Here's how the part is built. I have some questions about the finished solid (model axes, mm). Round coordinates to 2 decimals unless told otherwise and drop trailing zeros. Write each loop counter-clockwise with the first axis right and the second up, starting at its lowest first coordinate (ties: lowest second). Pieces come first, ordered by that corner, then holes. Notation, with made-up numbers: (56, -13) -> (75, -13) arc R21 ccw to (75, 11) -> close; hole circle Ø6 at (-36.75, -21). An arc over 180 degrees is marked (long way). Answer in a Markdown table with one row per item. Add a question column.
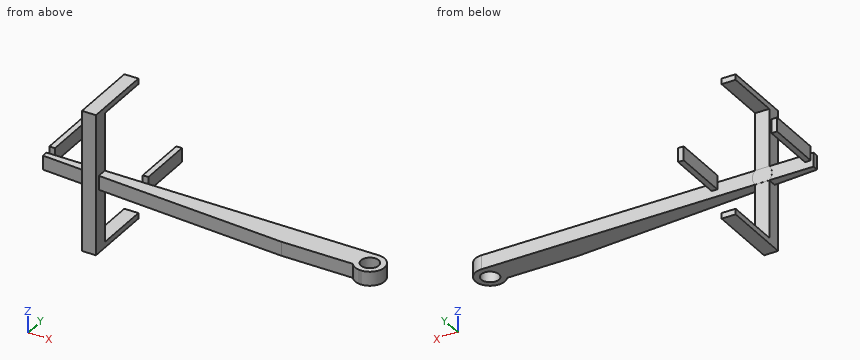
from build123d import *

# Parameters (mm, degrees)
SKETCH1_R             = 6.3
BOSS_EXTRUDE2_DEPTH   = 10
BODY_MOVE_COPY1_ANGLE = 90
BOSS_EXTRUDE4_DEPTH   = 10.5
BOSS_EXTRUDE5_DEPTH   = 0.05
SKETCH5_W             = 4
SKETCH5_H             = 39.958
BOSS_EXTRUDE6_DEPTH   = 10
SKETCH6_W             = 4
SKETCH6_H             = 40
BOSS_EXTRUDE7_DEPTH   = 10


# Read off the part's stored shape, not the designer's step: Boss-Extrude5
with BuildPart() as part:
    # Sketch1 → Boss-Extrude2 (new body)
    with BuildSketch(Plane.XY):
        with BuildLine():
            ThreePointArc((10.5, 0), (0, 10.5), (-10.5, 0))
            Line((-10.5, 0), (-10.5, -236.5))
            Line((-10.5, -236.5), (-6.3, -236.5))
            Line((-6.3, -236.5), (6.3, -59.125))
            Line((6.3, -59.125), (6.3, -8.4))
            ThreePointArc((6.3, -8.4), (9.035151526, -5.349395938), (10.394563839, -1.484265))
            Line((10.394563839, -1.484265), (10.5, 0))
        make_face()
        Circle(SKETCH1_R, mode=Mode.SUBTRACT)
    extrude(amount=BOSS_EXTRUDE2_DEPTH)


with BuildPart() as part_1:
    # Body-Move_Copy1: moved
    add(part.part.rotate(Axis((-34.8, -34.75, 0), (0, 0, -1)), BODY_MOVE_COPY1_ANGLE))


with BuildPart() as part_2:
    # Body-Move_Copy2: moved
    add(part_1.part.moved(Location((0, 69.6, 0))))

    # Sketch3 → Boss-Extrude4 (add)
    with BuildSketch(Plane(origin=(0, 0, 0), x_dir=(1, 0, 0), z_dir=(0, 1, 0))):
        Polygon((-195.05, 45), (-205.05, 45), (-205.05, -45), (-205.05, -55), (-195.05, -55), (-195.05, -5), align=None)
    extrude(amount=BOSS_EXTRUDE4_DEPTH)

    # Boss-Extrude5 outline → Boss-Extrude5 (add)
    with BuildSketch(Plane(origin=(0, 10.55, 0), x_dir=(1, 0, 0), z_dir=(0, 1, 0))):
        with BuildLine():
            ThreePointArc((-195.151020514, -10), (-193.05, -5), (-195.151020514, 0))
            Line((-195.151020514, 0), (-204.948979486, 0))
            ThreePointArc((-204.948979486, 0), (-207.05, -5), (-204.948979486, -10))
            Line((-204.948979486, -10), (-195.151020514, -10))
        make_face()
    extrude(amount=BOSS_EXTRUDE5_DEPTH)


with BuildPart() as part_3:
    # Body-Move_Copy4: moved
    add(part_2.part.moved(Location((0, 0, -5))))

    # Sketch5 → Boss-Extrude6 (add)
    with BuildSketch(Plane.XY.offset(10)):
        with Locations((-166.05, 30.529)):
            Rectangle(SKETCH5_W, SKETCH5_H)
        with Locations((-232.552850517, 30.529)):
            Rectangle(SKETCH5_W, SKETCH5_H)
    extrude(amount=-BOSS_EXTRUDE6_DEPTH)

    # Sketch6 → Boss-Extrude7 (add)
    with BuildSketch(Plane.ZY.offset(205.05)):
        with Locations((-48, 30.5)):
            Rectangle(SKETCH6_W, SKETCH6_H)
        with Locations((48, 30.5)):
            Rectangle(SKETCH6_W, SKETCH6_H)
    extrude(amount=-BOSS_EXTRUDE7_DEPTH)


solid = part_3.part
Item 1: For P1, Ø8, axis at x = -198.5, z = 5, coming from the -Y side; P2, Ø1.2, axis at x = -232, z = 8.5, coming from the -Y side; P3, Ø8, axis at y = 37, z = 3.5, coming from the +X side; P4, Ø10, axis at x = -100.5, y = 17, coming from the +Z side, each with a flat end and sliding along its axis, tell me the tip position at first contact or that it passes through.
Item 2: If we section it at C-C on x = -34: Please give me the cut outline in (y, z).
Item 3: If we section it at A-A on y = 32.5: Please give me the cut outline in (x, z).
Item 4: I need wall thicknesses on line 1 along Y through (x, z) = (0, 0); line 2 along X through (y, z) = (0.5, 33); line 3 along X through (y, z) = (33.5, 7). Which ranges of each line are inside material? Lowest first, please. Write a range as from..to.
Item 5: If we section it at B-B on z = 25.5: Please give me the cut outline in (x, y).
Results list:
| question | item | result |
|---|---|---|
| 1 | P1 | y = 0 |
| 1 | P2 | y = 10.55 |
| 1 | P3 | x = -164.05 |
| 1 | P4 | through |
| 2 | outline | (-6.25, -5) -> (10.55, -5) -> (10.55, 5) -> (-6.25, 5) -> close |
| 3 | outline | (-234.55, 0) -> (-230.55, 0) -> (-230.55, 10) -> (-234.55, 10) -> close; (-205.05, -50) -> (-195.05, -50) -> (-195.05, -46) -> (-205.05, -46) -> close; (-205.05, 46) -> (-195.05, 46) -> (-195.05, 50) -> (-205.05, 50) -> close; (-168.05, 0) -> (-164.05, 0) -> (-164.05, 10) -> (-168.05, 10) -> close |
| 4 | line 1 | -10.45..-6.25, 6.35..10.55 |
| 4 | line 2 | -205.05..-195.05 |
| 4 | line 3 | -234.55..-230.55, -168.05..-164.05 |
| 5 | outline | (-205.05, 0) -> (-195.05, 0) -> (-195.05, 10.5) -> (-205.05, 10.5) -> close |
